The listing builds one solid part. Answer for the finished solid, in the listing's coordinates (mm). Face numbers are marked on the shaded views. A direction names the side the tool comes from. Give positions to 0.01 mm unless a question says otherwise; leave off trailing zeros. Write each loop counter-clockwise with the first axis right and the second up, starting at its lowest first coordinate (ties: lowest second). Pieces come first, ordered by that corner, then holes. Notation, with made-up numbers: (4.25, -28) - (57.25, -28) arc R12 cw to (57.25, -6) - close; hole circle Ø7 at (-11, -6.5). An arc over 180 degrees is marked (long way). One line per item, written item: value. Start each with the question number.
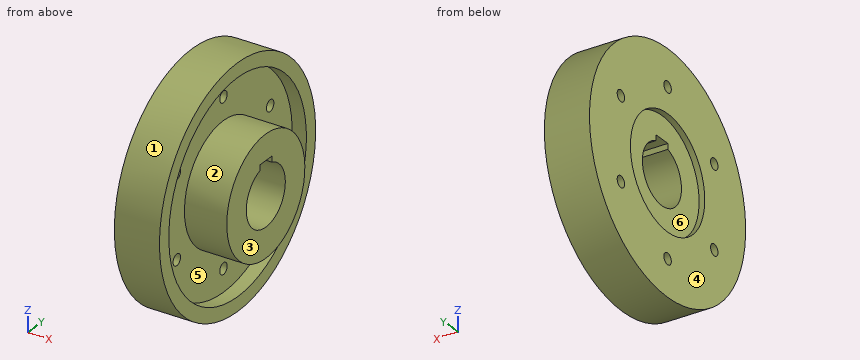
from build123d import *

# Parameters (mm, degrees)
SKETCH3_R               = 10
CUT_EXTRUDE1_DEPTH      = 307.30866785
CIRPATTERN1_COUNT       = 6
CUT_EXTRUDE2_DEPTH      = 325.191301549
CUT_EXTRUDE2_DEPTH_BACK = 325.191301549
SKETCH4_W               = 32
SKETCH4_H               = 10
CUT_EXTRUDE3_DEPTH      = 325.191301549
CUT_EXTRUDE3_DEPTH_BACK = 10
SKETCH5_R               = 100


with BuildPart() as part:
    # Sketch2 → Revolve1 (revolve)
    with BuildSketch(Plane(origin=(0, 0, 0), x_dir=(-1, 0, 0), z_dir=(0, 1, 0))):
        Polygon((-138.434782609, 52.5), (-268.434782609, 52.5), (-268.434782609, 105), (-193.434782609, 105), (-193.434782609, 185), (-218.434782609, 185), (-218.434782609, 210), (-138.434782609, 210), align=None)
    revolve(axis=Axis((0, 0, 0), (1, 0, 0)))

    # Sketch3 → Cut-Extrude1 (cut, through all)
    with BuildSketch(Plane.YZ.offset(193.434782609)):
        with Locations(Location((0, 145, 0), (0, 0, 270))):
            Circle(SKETCH3_R)
    cut_extrude1 = extrude(amount=-CUT_EXTRUDE1_DEPTH, mode=Mode.SUBTRACT)

    # CirPattern1: Cut-Extrude1 ×6 about axis
    cirpattern1_axis = Axis((0, 0, 0), (1, 0, 0))
    for i in range(1, CIRPATTERN1_COUNT):
        add(cut_extrude1.rotate(cirpattern1_axis, i * 360 / CIRPATTERN1_COUNT), mode=Mode.SUBTRACT)

    # Sketch4 → Cut-Extrude2 (cut, two sides: drawn at the far end of the back side and taken through both)
    with BuildSketch(Plane(origin=(138.434782609, 0, 0), x_dir=(0, -1, 0), z_dir=(-1, 0, 0)).offset(-CUT_EXTRUDE2_DEPTH_BACK)):
        with Locations((0, 55.002499938)):
            Rectangle(SKETCH4_W, SKETCH4_H)
    extrude(amount=CUT_EXTRUDE2_DEPTH + CUT_EXTRUDE2_DEPTH_BACK, mode=Mode.SUBTRACT)

    # Sketch5 → Cut-Extrude3 (cut, two sides: drawn at the far end of the back side and taken through both)
    with BuildSketch(Plane(origin=(138.434782609, 0, 0), x_dir=(0, -1, 0), z_dir=(-1, 0, 0)).offset(-CUT_EXTRUDE3_DEPTH_BACK)):
        with Locations(Location((0, 0, 0), (0, 0, 270))):
            Circle(SKETCH5_R)
    extrude(amount=CUT_EXTRUDE3_DEPTH + CUT_EXTRUDE3_DEPTH_BACK, mode=Mode.SUBTRACT)


solid = part.part
Item 1: Each of these flat-tipped pins is pushed along its axis until it touches: pin 1 Ø1.5 at (x, y) = (185.5, -123) entering from +Z; pin 2 Ø2 at (x, z) = (159, -95) entering from +Y; pin 3 Ø23 at (y, z) = (125.57, 72.5) entering from +X. Where does it stop, or does it pass through?
Item 2: Straight lines are drawn through the part: line 1 along Y through (x, z) = (209.25, 0); line 2 along Y through (x, z) = (187, 2.5); line 3 along Z through (x, y) = (150, 131.5). For each, find the intervals that lie inside material, in ascending order.
Item 3: For the marked faces 4, 5 and 6, determine the directions among +Z, -Z, +X, -X, +Y, -Y from which every point of the face is accessible in a straight line to the end or side of a thin tool.
Item 4: Find section B-B on z = 0. Determine the outline of the cut face in (x, y).
Item 5: Find section C-C on y = 0. Determine the outline of the cut face in (x, z).
Item 6: The mould has two halves that part along Y. Classify the marked faces 1, 2 and 3: +Y half, -Y half, draft (parallel to the pull), parting line (faces both ways), or undercut.
Item 7: Find section D-D on z = -72.5. Determine the outline of the cut face in (x, y), plus the area to 3 significant figures.
Item 8: Find section A-A on x = 211.5. Determine the outline of the cut face in (y, z).
Values:
1. pin 1: z = 170.75
1. pin 2: y = 187.79
1. pin 3: x = 193.43
2. line 1: -210 to -185, -105 to -52.5, 52.5 to 105, 185 to 210
2. line 2: -209.99 to -52.44, 52.44 to 209.99
2. line 3: -163.73 to -80.55, -64.45 to 64.45, 80.55 to 163.73
3. face 4: +Z, -Z, -X, +Y, -Y
3. face 5: +X
3. face 6: -X
4. outline: (138.43, -210) - (218.43, -210) - (218.43, -185) - (193.43, -185) - (193.43, -105) - (268.43, -105) - (268.43, -52.5) - (148.43, -52.5) - (148.43, -100) - (138.43, -100) - close; (138.43, 100) - (148.43, 100) - (148.43, 52.5) - (268.43, 52.5) - (268.43, 105) - (193.43, 105) - (193.43, 185) - (218.43, 185) - (218.43, 210) - (138.43, 210) - close
5. outline: (138.43, -210) - (218.43, -210) - (218.43, -185) - (193.43, -185) - (193.43, -155) - (138.43, -155) - close; (138.43, -135) - (193.43, -135) - (193.43, -105) - (268.43, -105) - (268.43, -52.5) - (148.43, -52.5) - (148.43, -100) - (138.43, -100) - close; (138.43, 100) - (148.43, 100) - (148.43, 60) - (268.43, 60) - (268.43, 105) - (193.43, 105) - (193.43, 135) - (138.43, 135) - close; (138.43, 155) - (193.43, 155) - (193.43, 185) - (218.43, 185) - (218.43, 210) - (138.43, 210) - close
6. face 1: parting line
6. face 2: undercut
6. face 3: draft
7. outline: (138.43, -197.09) - (218.43, -197.09) - (218.43, -170.2) - (193.43, -170.2) - (193.43, -135.57) - (138.43, -135.57) - close; (138.43, -115.57) - (193.43, -115.57) - (193.43, -75.95) - (268.43, -75.95) - (268.43, 75.95) - (193.43, 75.95) - (193.43, 115.57) - (138.43, 115.57) - (138.43, 68.87) - (148.43, 68.87) - (148.43, -68.87) - (138.43, -68.87) - close; (138.43, 135.57) - (193.43, 135.57) - (193.43, 170.2) - (218.43, 170.2) - (218.43, 197.09) - (138.43, 197.09) - close
7. area: 30,800 mm^2
8. outline: circle Ø420 at (0, 0); circle Ø210 at (0, 0); hole circle Ø370 at (0, 0); hole (-16, 50) arc R52.5 ccw (long way) to (16, 50) - (16, 60) - (-16, 60) - close
